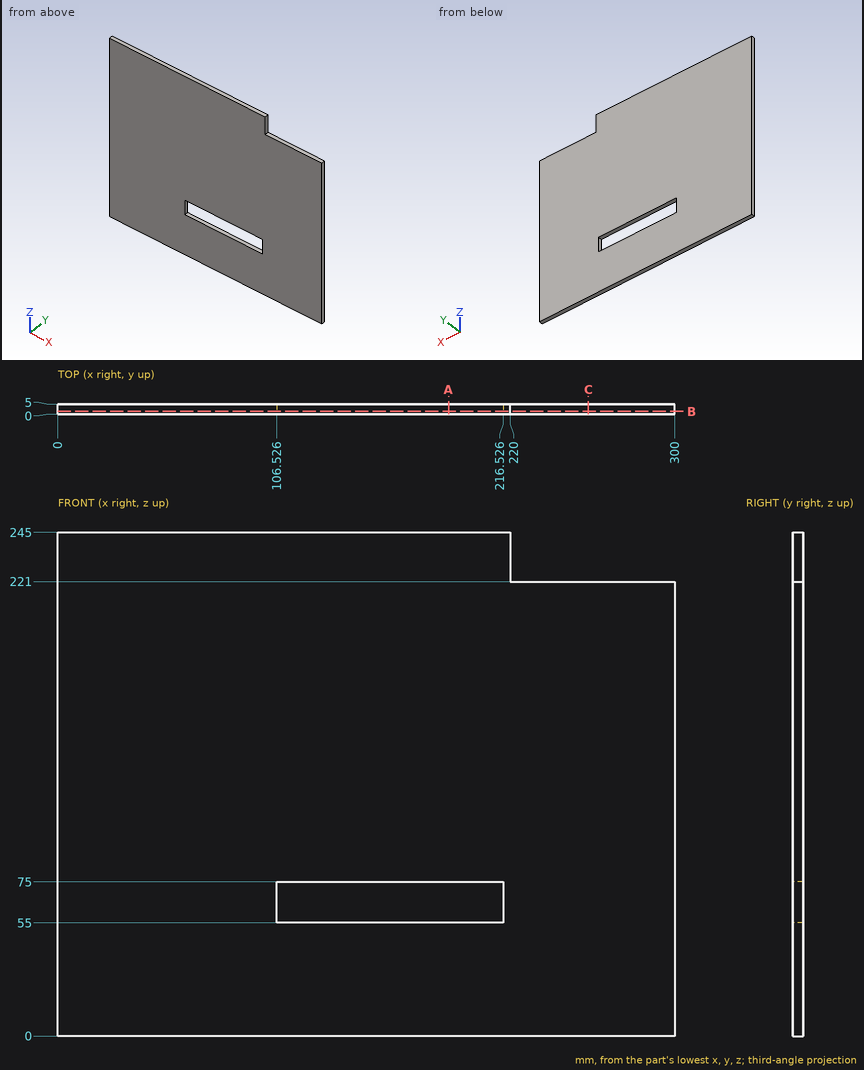
The figure shows three views and two pictorial views of one solid part (mm, origin at its lowest corner). Answer the questions. Give positions to 0.01 mm unless a question says otherwise; leave off trailing zeros. Order: outer loops, then holes, each group sorted by start corner. A loop starts at its lowest first (then second) coordinate and runs counter-clockwise, first axis right, second up. Notation, with made-up numbers: M -3,-29 L 39,-29 A21 ccw 39,-20 Z; hole C 12,60.25 d5. An arc over 180 degrees is marked long. Return JSON: item names as keys, results as strings.
1) Each of these flat-tipped pins is pushed along its axis until it touches: pin 1 (1.5 mm diameter, centred on y = 2.5, z = 227.5, fed in from +X); pin 2 (1.5 mm diameter, centred on y = 3, z = 62, fed in from -X). Where does it stop, or does it pass through?
Resolved:
{"pin 1": "x = 220", "pin 2": "x = 0"}
2) Section B-B, the plane y = 1.45 is taken. Write down the section's boundary in (x, z).
Resolved:
{"outline": "M 0,0 L 300,0 L 300,221 L 220,221 L 220,245 L 0,245 Z; hole M 106.53,55 L 216.53,55 L 216.53,75 L 106.53,75 Z"}
3) Straight lines are drawn through the part: line 1 along Z through (x, y) = (170.5, 4); line 2 along X through (y, z) = (1.15, 63.5); line 3 along Z through (x, y) = (255.5, 1.5). For each, find the intervals that lie inside material, in ascending order. Write a range as [from, to].
Resolved:
{"line 1": "[0, 55], [75, 245]", "line 2": "[0, 106.53], [216.53, 300]", "line 3": "[0, 221]"}
4) Section C-C, the plane x = 258 is taken. Write down the section's boundary in (y, z).
Resolved:
{"outline": "M 0,0 L 5,0 L 5,221 L 0,221 Z"}
5) Section A-A, the plane x = 190 is taken. Write down the section's boundary in (y, z), plus the area to 4 significant figures.
Resolved:
{"outline": "M 0,0 L 5,0 L 5,55 L 0,55 Z; M 0,75 L 5,75 L 5,245 L 0,245 Z", "area": "1,125 mm^2"}
